Work out the finished part from the listing and answer in its coordinate system (mm). Face numbers are marked on the shaded views. A direction names the side the tool comes from. Coordinates: 2 decimals unless noted, no trailing zeros. Order: outer loops, then holes, each group sorted by start corner. A loop starts at its lowest first (then second) coordinate and runs counter-clockwise, first axis right, second up. Notation, with made-up numbers: M 73.25,3.5 L 114.25,3.5 A10 cw 114.25,21.5 Z; hole C -33,48.5 d4. An arc over 180 degrees is marked long. Answer in a Markdown table with one row per item. Add a question column.
Item 1: The part is cut by section B-B (y = -44.5). Write down the section's boundary in (x, z).
Item 2: Which of the six approach directions +Z, -Z, +X, -X, +Y, -Y give full straight-line access (tool end or side, diameter ignored) to the marked faces 1, 2, 3 and 4?
Item 3: The part is cut by section C-C (z = -12.25). Write down the section's boundary in (x, y).
Item 4: Flat-ended cylindrical pins translate along their axes: pin 1 Ø15 at (y, z) = (-47.5, 4.5) entering from -X; pin 2 Ø1.5 at (x, z) = (14.5, 9.5) entering from -Y; pin 3 Ø9 at (y, z) = (-29.5, -0.5) entering from +X. Find the tip coordinate at first contact, or state that the pin passes through.
Item 5: The part is cut by section D-D (x = 20.5). Write down the section's boundary in (y, z), then the cut area to 3 significant figures.
Item 6: The part is cut by section A-A (z = 7). Write down the section's boundary in (x, y).
Item 7: The mould has two halves that part along Y. Classify the marked faces 5, 6 and 7: released by +Y, released by -Y, zero draft, split by the parting line, or undercut.
Item 8: Consider line 1 (Y direction, x = 0, z = -10.5); line 2 (X direction, y = -3.5, z = 7.25); line 3 (X direction, y = -39, z = 3.5). Determine where each line is inside the solid, lowest interval first. Write a range as from..to.
from build123d import *

# Parameters (mm, degrees)
BOSS_EXTRUDE1_DEPTH = 15
CUT_EXTRUDE1_DEPTH  = 12
CUT_EXTRUDE2_REACH  = 81.096
SKETCH3_R           = 10


with BuildPart() as part:
    # Sketch1 → Boss-Extrude1 (new body)
    with BuildSketch(Plane.XY):
        with BuildLine():
            Line((-7.5, 0), (-7.5, -65))
            Line((-7.5, -65), (-15, -65))
            Line((-15, -65), (-15, -42.295968202))
            Line((-15, -42.295968202), (-15, -34.378221735))
            ThreePointArc((-15, -34.378221735), (-15.681483474, -29.201840833), (-17.679491924, -24.378221735))
            Line((-17.679491924, -24.378221735), (-23.815698604, -13.75))
            ThreePointArc((-23.815698604, -13.75), (0, 27.5), (23.815698604, -13.75))
            Line((23.815698604, -13.75), (17.679491924, -24.378221735))
            ThreePointArc((17.679491924, -24.378221735), (15.681483474, -29.201840833), (15, -34.378221735))
            Line((15, -34.378221735), (15, -65))
            Line((15, -65), (7.5, -65))
            Line((7.5, -65), (7.5, 0))
            ThreePointArc((7.5, 0), (0, 7.5), (-7.5, 0))
        make_face()
    extrude(amount=BOSS_EXTRUDE1_DEPTH)

    # Sketch2 → Cut-Extrude1 (cut)
    with BuildSketch(Plane.XY.offset(15)):
        with BuildLine():
            Line((-12.5, 0), (-12.5, -12.153212483))
            ThreePointArc((-12.5, -12.153212483), (-14.723542865, -15.050989962), (-18.098076211, -13.653212483))
            Line((-18.098076211, -13.653212483), (-19.485571585, -11.25))
            ThreePointArc((-19.485571585, -11.25), (0, 22.5), (19.485571585, -11.25))
            Line((19.485571585, -11.25), (18.098076211, -13.653212483))
            ThreePointArc((18.098076211, -13.653212483), (14.723542865, -15.050989962), (12.5, -12.153212483))
            Line((12.5, -12.153212483), (12.5, 0))
            ThreePointArc((12.5, 0), (0, 12.5), (-12.5, 0))
        make_face()
    extrude(amount=-CUT_EXTRUDE1_DEPTH, mode=Mode.SUBTRACT)

    # Mirror1: part across plane


with BuildPart() as part_1:
    add(part.part)
    add(part.part.mirror(Plane.XY))

    # Sketch3 → Cut-Extrude2 (cut, up to next)
    with BuildSketch(Plane(origin=(15, 0, 0), x_dir=(0, 0, -1), z_dir=(1, 0, 0)), mode=Mode.PRIVATE) as cut_extrude2_sk1:
        with BuildLine():
            Line((15, -65), (15, -50))
            ThreePointArc((15, -50), (10.606601718, -60.606601718), (0, -65))
            Line((0, -65), (15, -65))
        make_face()
    cut_extrude2_tool1 = extrude(cut_extrude2_sk1.sketch, amount=-CUT_EXTRUDE2_REACH, mode=Mode.PRIVATE) & part_1.part
    # Sketch3 → Cut-Extrude2 (cut, up to next)
    with BuildSketch(Plane(origin=(15, 0, 0), x_dir=(0, 0, -1), z_dir=(1, 0, 0)), mode=Mode.PRIVATE) as cut_extrude2_sk2:
        with BuildLine():
            ThreePointArc((0, -65), (-10.606601718, -60.606601718), (-15, -50))
            Line((-15, -50), (-15, -65))
            Line((-15, -65), (0, -65))
        make_face()
    cut_extrude2_tool2 = extrude(cut_extrude2_sk2.sketch, amount=-CUT_EXTRUDE2_REACH, mode=Mode.PRIVATE) & part_1.part
    # Sketch3 → Cut-Extrude2 (cut, up to next)
    with BuildSketch(Plane(origin=(15, 0, 0), x_dir=(0, 0, -1), z_dir=(1, 0, 0)), mode=Mode.PRIVATE) as cut_extrude2_sk3:
        with Locations((0, -50)):
            Circle(SKETCH3_R)
    cut_extrude2_tool3 = extrude(cut_extrude2_sk3.sketch, amount=-CUT_EXTRUDE2_REACH, mode=Mode.PRIVATE) & part_1.part
    cut_extrude2_1 = cut_extrude2_tool1.solids().sort_by_distance((15, -61.649481, -11.649481))[0]
    add(cut_extrude2_1, mode=Mode.SUBTRACT)
    cut_extrude2_2 = cut_extrude2_tool2.solids().sort_by_distance((15, -61.649481, 11.649481))[0]
    add(cut_extrude2_2, mode=Mode.SUBTRACT)
    cut_extrude2_3 = cut_extrude2_tool3.solids().sort_by_distance((15, -50, 0))[0]
    add(cut_extrude2_3, mode=Mode.SUBTRACT)
    cut_extrude2 = cut_extrude2_1 + cut_extrude2_2 + cut_extrude2_3  # Cut-Extrude2 as one shape, for the pattern or mirror that repeats it

    # Mirror2: Cut-Extrude2 across plane
    add(cut_extrude2.mirror(Plane(origin=(0, 0, 0), x_dir=(0, 0, 1), z_dir=(1, 0, 0))), mode=Mode.SUBTRACT)


solid = part_1.part
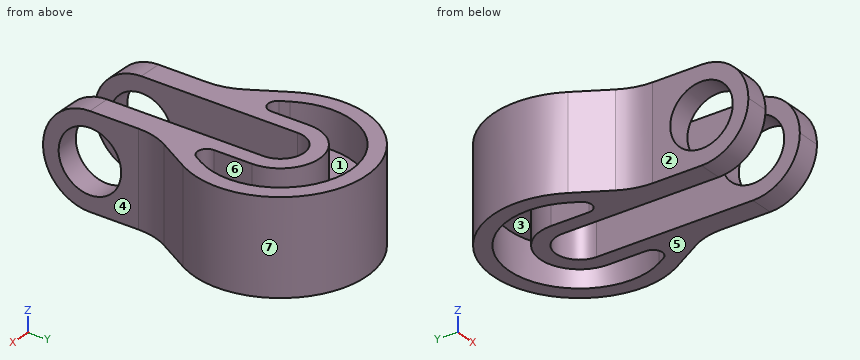
Reply:
| question | item | result |
|---|---|---|
| 1 | outline | M -15,-15 L -7.5,-15 L -7.5,-8.35 L -15,-8.35 Z; M -15,8.35 L -7.5,8.35 L -7.5,15 L -15,15 Z; M 7.5,-15 L 15,-15 L 15,-8.35 L 7.5,-8.35 Z; M 7.5,8.35 L 15,8.35 L 15,15 L 7.5,15 Z |
| 2 | face 1 | +Z |
| 2 | face 2 | +Z, -Z, -X, -Y |
| 2 | face 3 | -Z |
| 2 | face 4 | +Z, -Z, +X, -Y |
| 3 | outline | M -23.82,-13.75 L -17.68,-24.38 A20 cw -15,-34.38 L -15,-58.66 L -7.5,-58.66 L -7.5,0 A7.5 cw 7.5,0 L 7.5,-58.66 L 15,-58.66 L 15,-34.38 A20 cw 17.68,-24.38 L 23.82,-13.75 A27.5 ccw long Z; hole M -19.49,-11.25 L -18.1,-13.65 A3 ccw -12.5,-12.15 L -12.5,0 A12.5 cw 12.5,0 L 12.5,-12.15 A3 ccw 18.1,-13.65 L 19.49,-11.25 A22.5 ccw long Z |
| 4 | pin 1 | stops at x = -15 |
| 4 | pin 2 | stops at y = -62.18 |
| 4 | pin 3 | stops at x = 17.34 |
| 5 | outline | M -19.49,-15 L -9.27,-15 L -9.27,-3 L 9.27,-3 L 9.27,-15 L 18.33,-15 L 18.33,15 L 9.27,15 L 9.27,3 L -9.27,3 L -9.27,15 L -19.49,15 Z |
| 5 | area | 690 mm2 |
| 6 | outline | M -23.82,-13.75 L -17.68,-24.38 A20 cw -15,-34.38 L -15,-42.86 L -7.5,-42.86 L -7.5,0 A7.5 cw 7.5,0 L 7.5,-42.86 L 15,-42.86 L 15,-34.38 A20 cw 17.68,-24.38 L 23.82,-13.75 A27.5 ccw long Z; M -15,-63.27 L -7.5,-63.27 L -7.5,-57.14 L -15,-57.14 Z; M 7.5,-63.27 L 15,-63.27 L 15,-57.14 L 7.5,-57.14 Z; hole M -19.49,-11.25 L -18.1,-13.65 A3 ccw -12.5,-12.15 L -12.5,0 A12.5 cw 12.5,0 L 12.5,-12.15 A3 ccw 18.1,-13.65 L 19.49,-11.25 A22.5 ccw long Z |
| 7 | face 5 | zero draft |
| 7 | face 6 | undercut |
| 7 | face 7 | split by the parting line |
| 8 | line 1 | y = 7.5..12.5, 22.5..27.5 |
| 8 | line 2 | x = -27.28..-22.23, -12.5..-7.5, 7.5..12.5, 22.23..27.28 |
| 8 | line 3 | x = -15..-7.5, 7.5..15 |
